Geometry: final body of the model. Coordinates: model frame, mm. A direction names the side the tool comes from. Coordinates: 2 decimals unless noted, no trailing zeros. Write each loop counter-clockwise with the first axis right and the second up, starting at its lowest first coordinate (ties: lowest second). Pieces come first, ordered by that corner, then holes. Notation, with made-up numbers: (3.25, -18) -> (12.25, -18) arc R36 ccw to (12.25, 19) -> close; hole circle Ø7 at (43.25, 17.25). An arc over 180 degrees is marked (long way). Answer as a JSON object with one key per item and string values. Group by question number.
Solid Edge part; units mm, degrees
sketch "Sketch1" plane through (0, 0, 0) normal (0, -1, 0) x (1, 0, 0)
  circle A0 centre (0, 0) radius 10
extrude "Extrusionsausprägung_15" add sketch "Sketch1" along normal blind 150
sketch "Sketch2" plane through (0, -136, 0) normal (0, -1, 0) x (-1, 0, 0)
  line L0 (42.474, 10.1) -> (-42.474, 10.1)
  line L1 (-42.474, 10.1) -> (-42.474, 8.1)
  line L2 (-42.474, 8.1) -> (42.474, 8.1)
  line L3 (42.474, 8.1) -> (42.474, 10.1)
extrude "Extrusionsausschnitt_23" cut sketch "Sketch2" along normal mid plane 29
sketch "Sketch3" plane through (0, -76, 0) normal (0, -1, 0) x (-1, 0, 0)
  line L0 (-42.474, 10.1) -> (42.474, 10.1)
  line L1 (42.474, 10.1) -> (42.474, 8.1)
  line L2 (42.474, 8.1) -> (-42.474, 8.1)
  line L3 (-42.474, 8.1) -> (-42.474, 10.1)
extrude "Extrusionsausprägung_16" cut sketch "Sketch3" along normal mid plane 12
sketch "Sketch4" plane through (0, -42, 0) normal (0, -1, 0) x (-1, 0, 0)
  line L0 (-42.474, 10.1) -> (42.474, 10.1)
  line L1 (42.474, 10.1) -> (42.474, 8.1)
  line L2 (42.474, 8.1) -> (-42.474, 8.1)
  line L3 (-42.474, 8.1) -> (-42.474, 10.1)
extrude "Extrusionsausschnitt_25" cut sketch "Sketch4" along normal mid plane 12
Item 1: Contact query for flat-ended pins moving along their axis: pin 1 (1 mm diameter, centred on x = 0, z = -9.5, fed in from -Y); pin 2 (1.5 mm diameter, centred on x = 2.5, y = -91, fed in from -Z); pin 3 (1 mm diameter, centred on y = -45.5, z = 6, fed in from +X). Output: stop coordinate, or through.
Item 2: Set-up query: faces 5 (the flat face through (0, -136, -8.1)), 6 (the flat face through (0, -150, 1)). Return all of +Z, -Z, +X, -X, +Y, -Y with unobstructed straight access to the full face (end or side cutting, diameter ignored); none if empty.
Item 3: Section C-C on z = 2. Output: boundary loops of the cut face in (x, y).
Item 4: Section D-D on x = 8. Output: boundary loops of the cut face in (y, z).
Item 5: Mould query, pull axis Y, two halves, no side actions, for faces 1 (the flat face through (0, -42, -8.1)), 2 (the flat face through (0, 0, 0)), 3 (the cylindrical face through (-2.17, -73.95, 9.76)), 4 (the flat face through (0, -76, -8.1)). Classes: +Y half, -Y half, draft (parallel to the pull), parting line (faces both ways), or undercut.
Item 6: Section B-B on y = -137. Output: boundary loops of the cut face in (x, z).
Item 7: Ray query, L1, parallel to Y at x = 4, z = -8.75; L2, parallel to Z at x = 0.25, y = -92.5; L3, parallel to X at y = -105.5, z = 8.5. Return the intervals inside material, ascending. Write a range as [from, to].
Item 8: Section A-A on x = 0. Output: boundary loops of the cut face in (y, z), then the cut area to 3 significant figures.
Answer sheet:
{
 "1": {"pin 1": "stops at y = -121.5", "pin 2": "stops at z = -9.85", "pin 3": "stops at x = 8.35"},
 "2": {"face 5": "-Z, +X, -X, -Y", "face 6": "+Z, -Z, +X, -X, -Y"},
 "3": {"outline": "(-9.8, -150) -> (9.8, -150) -> (9.8, 0) -> (-9.8, 0) -> close"},
 "4": {"outline": "(-150, -6) -> (0, -6) -> (0, 6) -> (-150, 6) -> close"},
 "5": {"face 1": "undercut", "face 2": "+Y half", "face 3": "draft", "face 4": "undercut"},
 "6": {"outline": "(-5.86, -8.1) -> (5.86, -8.1) arc R10 ccw (long way) to start"},
 "7": {"L1": "y = [-121.5, -82], [-70, -48], [-36, 0]", "L2": "z = [-10, 10]", "L3": "x = [-5.27, 5.27]"},
 "8": {"outline": "(-150, -8.1) -> (-121.5, -8.1) -> (-121.5, -10) -> (-82, -10) -> (-82, -8.1) -> (-70, -8.1) -> (-70, -10) -> (-48, -10) -> (-48, -8.1) -> (-36, -8.1) -> (-36, -10) -> (0, -10) -> (0, 10) -> (-150, 10) -> close", "area": "2,900 mm^2"}
}
